Geometry: see drawing. Coordinates: mm, zero at the bounding-box minimum. A direction names the side the tool comes from. Give positions to 0.01 mm unless a question says otherwise; leave off trailing zeros. Order: outer loops, then holes, each group sorted by start corner. A loop starts at its lowest first (then second) coordinate and runs counter-clockwise, first axis right, second up. Notation, with made-up numbers: (56, -13.75) - (115, -13.75) arc R32 ccw to (115, 18.25) - close; hole circle Ø9 at (33, -37). An arc over 180 degrees is marked (long way). Put each result on its own line as item: value. Start each with the question number.
1. Mould query, pull axis Z, two halves, no side actions, for the marked faces 1, 2 and 3. Classes: pulls with the +Z half, pulls with the -Z half, needs draft (parallel to the pull), parting line crosses it, or undercut.
2. First-contact query: P1, Ø3, axis at y = 22.5, z = 41, coming from the -X side; P2, Ø1.4, axis at x = 21.5, y = 40, coming from the +Z side; P3, Ø4.5, axis at y = 10, z = 20, coming from the -X side. Flat tips, straight axial feed; report the tip coordinate or a pass-through.
3. Section A-A on x = 8.5. Return the cut outline in (y, z) (1 decimal).
4. Ray query, line 1 along Y through (x, z) = (21.5, 35); line 2 along Y through (x, z) = (21.5, 43); line 3 along X through (y, z) = (10, 40.25). Return the intervals inside material, ascending. Write a range as from..to.
5. Section B-B on y = 19.5. Return the cut outline in (x, z).
6. Set-up query: the marked faces 4 and 5. Return all of +Z, -Z, +X, -X, +Y, -Y with unobstructed straight access to the full face (end or side cutting, diameter ignored); none if empty.
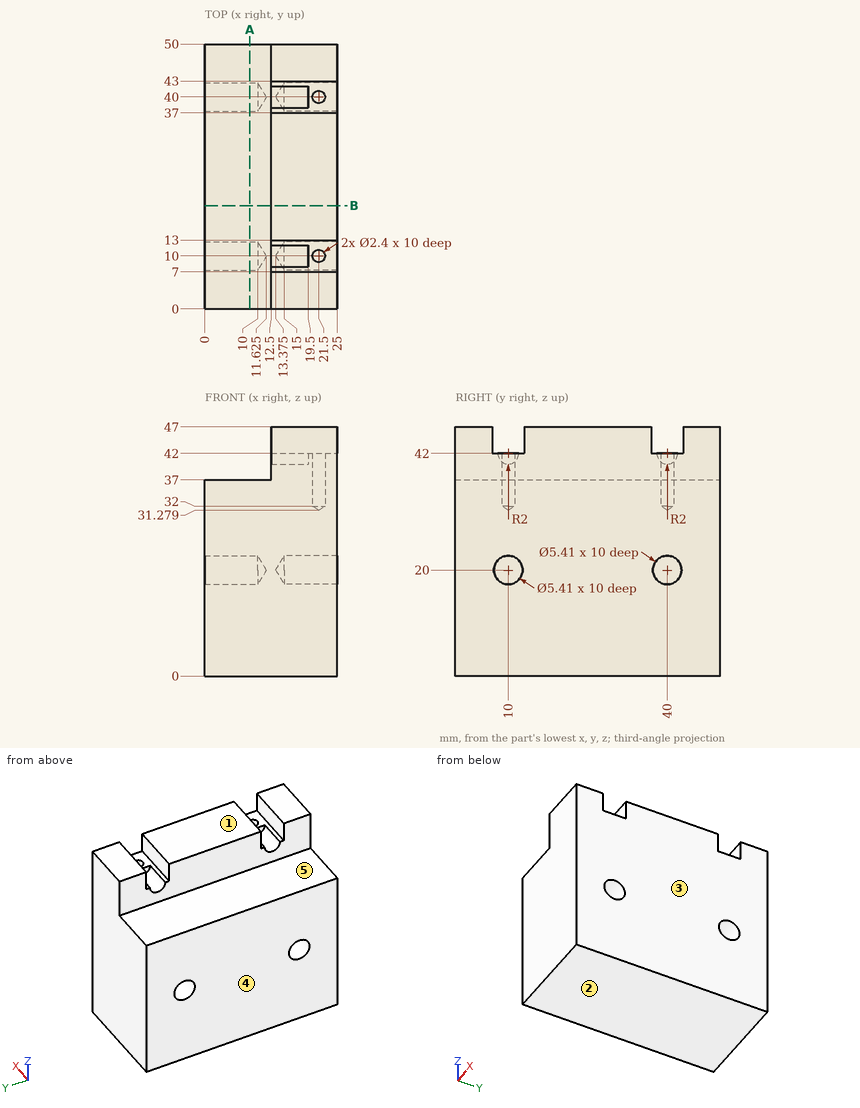
Resolved:
1. face 1: pulls with the +Z half
1. face 2: pulls with the -Z half
1. face 3: needs draft
2. P1: x = 12.5
2. P2: z = 31.7
2. P3: x = 10.27
3. outline: (0, 0) - (50, 0) - (50, 37) - (0, 37) - close; hole circle Ø5.4 at (10, 20); hole circle Ø5.4 at (40, 20)
4. line 1: 0..8.8, 11.2..38.8, 41.2..50
4. line 2: 0..7, 13..37, 43..50
4. line 3: 19.5..20.3, 22.7..25
5. outline: (0, 0) - (25, 0) - (25, 47) - (12.5, 47) - (12.5, 37) - (0, 37) - close
6. face 4: +Z, -Z, -X, +Y, -Y
6. face 5: +Z, -X, +Y, -Y
